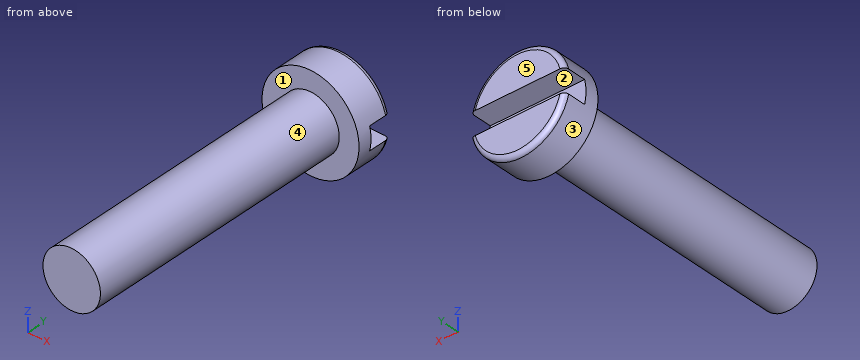
Autodesk Inventor part; units mm, degrees
ref_plane "YZ Plane" through (0, 0, 0) normal (1, 0, 0) x (0, 1, 0)
ref_plane "XZ Plane" through (0, 0, 0) normal (0, 1, 0) x (-1, 0, 0)
ref_plane "XY Plane" through (0, 0, 0) normal (0, 0, 1) x (1, 0, 0)
sketch "Sketch1" plane through (0, 0, 0) normal (0, 1, 0) x (-1, 0, 0)
  circle A0 centre (0, 0) radius 2.5
  dimension "d0" = 5
extrude "Extrusion1" add sketch "Sketch1" along normal blind 24
sketch "Sketch2" plane through (0, 24, 0) normal (0, 1, 0) x (1, 0, 0)
  circle A0 centre (0, 0) radius 4.225
  dimension "d3" = 8.45
extrude "Extrusion2" add sketch "Sketch2" along normal blind 3.2
sketch "Sketch3" plane through (0, 27.2, 0) normal (0, 1, 0) x (1, 0, 0)
  line L0 (-5, -1) -> (5, -1)
  line L1 (5, -1) -> (5, 1)
  line L2 (5, 1) -> (-5, 1)
  line L3 (-5, 1) -> (-5, -1)
  point P0 (0, 0)
  dimension "d6" = 10
  dimension "d7" = 2
  dimension "d8" = 5
  dimension "d9" = 1
extrude "Extrusion3" cut sketch "Sketch3" against normal blind 2
fillet "Fillet1" radius 0.4 2 edges at (0, 27.2, 4.225) (0, 27.2, -4.225)
properties part number "machine_screw_5_x_24_mm"
Can you work these out from the model? Positions are in its coordinate system, mm. Face numbers are marked on the shaded views. A direction names the side the tool comes from. Round coordinates to 2 decimals unless told otherwise and drop trailing zeros. Loops run counter-clockwise (first coordinate to the right, second up) from the corner with the lowest first, then second, coordinate; pieces in that order, holes last. Notation, with made-up numbers: (87.25, 3) - (130.25, 3) arc R30 cw to (130.25, 27) - close; hole circle Ø3 at (-20.75, -5). An arc over 180 degrees is marked (long way). Answer in a Markdown table with one row per item. Add a question column.
Q1. I want a section at C-C on y = 23. List the corners of the cut face in (x, z) for me.
Q2. Which directions (+Z, -Z, +X, -X, +Y, -Y) give clear straight access to the entire face, cutting with the end or side of a thin tool? Please do the marked faces 4 and 5.
Q3. I want a section at B-B on z = 0. List the corners of the cut face in (x, y) for me (3 decimals), and give its area (3 significant figures).
Q4. I need wall thicknesses on L1, parallel to Y at x = -1, z = -3.25; L2, parallel to Y at x = 2.75, z = -0.5; L3, parallel to X at y = 9.5, z = -0.5. Which ranges of each line are inside material? Lowest first, please.
Q5. I want a section at A-A on x = 0. List the corners of the cut face in (y, z) for me (3 decimals).
Q6. For pin 1 Ø1 at (x, y) = (1.5, 26.5) entering from -Z; pin 2 Ø5 at (x, y) = (0.5, 4.5) entering from +Z; pin 3 Ø1.6 at (x, y) = (1.5, 26.5) entering from +Z, each with a flat end and sliding along its axis, tell me the tip position at first contact or that it passes through.
Q7. We'd pull the mould along Z, two halves only. Please class the marked faces 1, 2 and 3: pulls with the +Z half, pulls with the -Z half, needs draft (parallel to the pull), parting line crosses it, or undercut.
A:
| question | item | result |
|---|---|---|
| 1 | outline | circle Ø5 at (0, 0) |
| 2 | face 4 | -Y |
| 2 | face 5 | +Z, -Z, +X, -X, +Y |
| 3 | outline | (-4.225, 24) - (-2.5, 24) - (-2.5, 0) - (2.5, 0) - (2.5, 24) - (4.225, 24) - (4.225, 25.2) - (-4.225, 25.2) - close |
| 3 | area | 130 mm^2 |
| 4 | L1 | 24 to 27.2 |
| 4 | L2 | 24 to 25.2 |
| 4 | L3 | -2.45 to 2.45 |
| 5 | outline | (0, -2.5) - (24, -2.5) - (24, -4.225) - (26.8, -4.225) arc R0.4 ccw to (27.2, -3.825) - (27.2, -1) - (25.2, -1) - (25.2, 1) - (27.2, 1) - (27.2, 3.825) arc R0.4 ccw to (26.8, 4.225) - (24, 4.225) - (24, 2.5) - (0, 2.5) - close |
| 6 | pin 1 | z = -4.1 |
| 6 | pin 2 | z = 2.5 |
| 6 | pin 3 | z = 4.17 |
| 7 | face 1 | needs draft |
| 7 | face 2 | undercut |
| 7 | face 3 | parting line crosses it |
